The figure shows three views and two pictorial views of one solid part (mm, origin at its lowest corner). Answer the questions. Coordinates: 2 decimals unless noted, no trailing zeros. Order: outer loops, then holes, each group sorted by start corner. A loop starts at its lowest first (then second) coordinate and runs counter-clockwise, first axis right, second up. Notation, with made-up numbers: (79.5, 1) -> (130.5, 1) arc R20 cw to (130.5, 22) -> close; hole circle Ø9 at (45, 58). An arc over 180 degrees is marked (long way). Return JSON: item names as keys, results as strings.
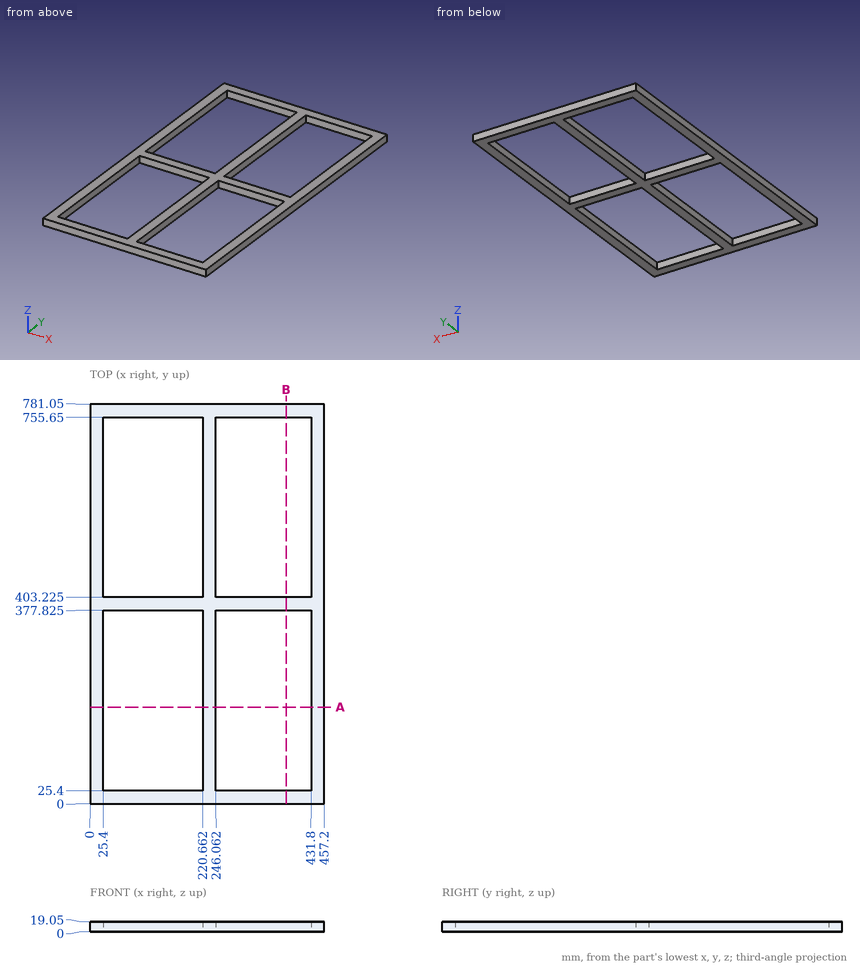
Item 1: The part is cut by section B-B on x = 383. Count the separate pieces of the cut face and the enclosed holes in it, plus the area to 3 significant figures.
Answer list:
{"separate pieces": "3", "enclosed holes": "0", "area": "1,450 mm2"}
Item 2: Find the intervals of material crossed by probe 1 along X at (y, z) = (166.5, 2.25), in increasing order.
Answer list:
{"probe 1": "0 to 25.4, 220.66 to 246.06, 431.8 to 457.2"}
Item 3: The part is cut by section A-A on y = 189. Determine the outline of the cut face in (x, z).
Answer list:
{"outline": "(0, 0) -> (25.4, 0) -> (25.4, 19.05) -> (0, 19.05) -> close; (220.66, 0) -> (246.06, 0) -> (246.06, 19.05) -> (220.66, 19.05) -> close; (431.8, 0) -> (457.2, 0) -> (457.2, 19.05) -> (431.8, 19.05) -> close"}
